Autodesk Inventor part; units mm, degrees
ref_plane "YZ Plane" through (0, 0, 0) normal (1, 0, 0) x (0, 1, 0)
ref_plane "XZ Plane" through (0, 0, 0) normal (0, 1, 0) x (-1, 0, 0)
ref_plane "XY Plane" through (0, 0, 0) normal (0, 0, 1) x (1, 0, 0)
sketch "Esquisse1" plane through (0, 0, 0) normal (0, 0, 1) x (1, 0, 0)
  line L0 (0, 21) -> (40, 21)
  line L1 (40, 21) -> (40, 0)
  line L2 (40, 0) -> (0, 0)
  line L3 (0, 0) -> (0, 21)
  line L4 (-8, 0) -> (48, 0)
  line L5 (0, -4.2) -> (0, 25.2)
  point P0 (0, 0)
  dimension "d0" = 40
  dimension "d1" = 21
extrude "Extrusion1" add sketch "Esquisse1" along normal mid plane 76
sketch "Esquisse2" plane through (0, 0, 38) normal (0, 0, 1) x (1, 0, 0)
  circle A0 centre (10, 10.5) radius 7
  circle A1 centre (30, 10.5) radius 7
  line L0 (40, 21) -> (0, 21)
  line L1 (0, 21) -> (0, 0)
  line L2 (40, 0) -> (40, 21)
  line L3 (0, 0) -> (40, 0)
  dimension "d4" = 14
  dimension "d5" = 14
  dimension "d11" = 10.5
  dimension "d20" = 10.5
  dimension "d21" = 20
extrude "Extrusion2" cut sketch "Esquisse2" against normal through all contours A0 | A1
sketch "Esquisse3" plane through (0, 21, 38) normal (0, 1, 0) x (1, 0, 0)
  line L0 (2, 74) -> (38, 74)
  line L1 (38, 74) -> (38, 2)
  line L2 (38, 2) -> (2, 2)
  line L3 (2, 2) -> (2, 74)
  line L4 (0, 76) -> (40, 76)
  line L5 (40, 0) -> (0, 0)
  line L6 (40, 76) -> (40, 0)
  line L7 (0, 76) -> (0, 0)
  point P0 (0, 38)
  dimension "d14" = 2
  dimension "d15" = 2
  dimension "d16" = 2
  dimension "d17" = 2
extrude "Extrusion3" cut sketch "Esquisse3" against normal blind 14 contours L0 L1 L2 L3
sketch "Esquisse4" plane through (0, 7, 38) normal (0, 1, 0) x (1, 0, 0)
  line L0 (2, 74) -> (19, 74)
  line L1 (19, 74) -> (19, 2)
  line L2 (19, 2) -> (2, 2)
  line L3 (2, 2) -> (2, 74)
  line L4 (20.5, 74) -> (38, 74)
  line L5 (38, 74) -> (38, 2)
  line L6 (38, 2) -> (20.5, 2)
  line L7 (20.5, 2) -> (20.5, 74)
  line L8 (2, 74) -> (38, 74)
  line L9 (2, 2) -> (2, 74)
  line L10 (38, 74) -> (38, 2)
  line L11 (38, 2) -> (2, 2)
  point P0 (0, 38)
  dimension "d22" = 1.5
  dimension "d23" = 17
extrude "Extrusion4" cut sketch "Esquisse4" against normal blind 5 contours L0 L1 L2 L3 | L4 L5 L6 L7
sketch "Esquisse5" plane through (0, 0, 38) normal (0, -1, 0) x (1, 0, 0)
  line L0 (0, 0) -> (40, 0)
  line L1 (0, 0) -> (0, -76)
  line L2 (40, -76) -> (40, 0)
  line L3 (40, -76) -> (0, -76)
  point P0 (0, -38)
  point P1 (10, -10)
  point P2 (10, -38)
  point P3 (30, -38)
  point P4 (30, -66)
  point P5 (30, -10)
  point P6 (10, -66)
  dimension "d26" = 28
  dimension "d27" = 28
  dimension "d28" = 10
  dimension "d29" = 10
  dimension "d30" = 10
  dimension "d31" = 10
  dimension "d32" = 20
  dimension "d33" = 38
  dimension "d41" = 28
  dimension "d42" = 28
  dimension "d43" = 20
hole "Perçage1" at (10, 0, 28) at (10, 0, 0) at (30, 0, 0) at (30, 0, -28) at (10, 0, -28) at (30, 0, 28) direction (0, 1, 0) diameter 2 end through all
equation "\"d5\" = d4"
equation "\"d11\" = d20"
equation "\"d15\" = d14"
equation "\"d16\" = d15"
equation "\"d17\" = d16"
properties part number "support pile"
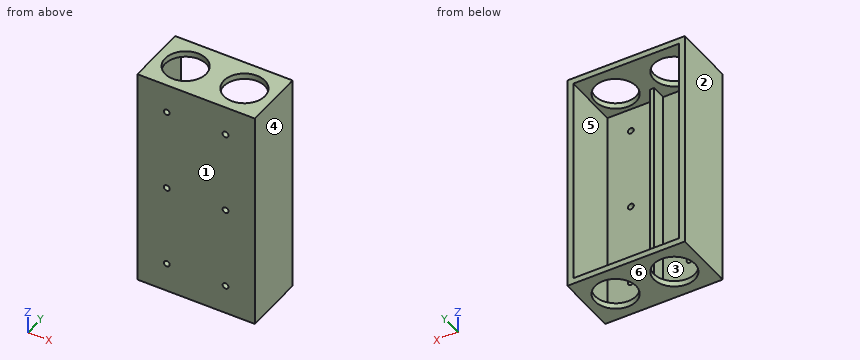
Design review of the part built by this model. Coordinates are the model's own, in mm. Face numbers are marked on the shaded views. A direction names the side the tool comes from. Round coordinates to 2 decimals unless told otherwise and drop trailing zeros. Write each loop counter-clockwise with the first axis right and the second up, starting at its lowest first coordinate (ties: lowest second). Pieces come first, ordered by that corner, then holes.
Item 1: We need section B-B on x = 10. Write out the cut boundary in (y, z).
Item 2: Clearance check with flat-ended pins moving along their axes: pin 1 Ø13.5 at (x, z) = (11, 0) entering from +Y; pin 2 Ø2.5 at (x, z) = (10, 0) entering from -Y; pin 3 Ø19 at (x, z) = (27, 1) entering from +Y. State where each tip first meets the part, or that it passes through.
Item 3: For probe 1 along X at (y, z) = (1.5, -28); probe 2 along X at (y, z) = (5.5, 30.5); probe 3 along Z at (x, y) = (30, 1.25), list the stretches that pass through material, from the lowest coordinate up.
Item 4: We need section A-A on z = 28. Write out the cut boundary in (x, y).
Item 5: We need section D-D on y = 6.25. Write out the cut boundary in (x, z), and give its area (3 significant figures).
Item 6: For the marked faces 5 and 6, list the 3-axis set-ups (+Z, -Z, +X, -X, +Y, -Y) from which the entire face can be reached by the end or side of a thin tool; tool diameter is ignored.
Item 7: We need section C-C on y = 10.5. Write out the cut boundary in (x, z), and give its area (3 significant figures).
Item 8: The part is to be moulded in two halves that separate along X. For the marked faces 1, 2, 3 and 4, say which applies: +X half, -X half, draft (parallel to the pull), parting line (faces both ways), or undercut.
Returned:
1. outline: (0, -38) - (3.5, -38) - (3.5, -36) - (2, -36) - (2, -29) - (0, -29) - close; (0, -27) - (2, -27) - (2, -1) - (0, -1) - close; (0, 1) - (2, 1) - (2, 27) - (0, 27) - close; (0, 29) - (2, 29) - (2, 36) - (3.5, 36) - (3.5, 38) - (0, 38) - close; (17.5, -38) - (21, -38) - (21, -36) - (17.5, -36) - close; (17.5, 36) - (21, 36) - (21, 38) - (17.5, 38) - close
2. pin 1: stops at y = 2
2. pin 2: stops at y = 0
2. pin 3: stops at y = 7
3. probe 1: x = 0 to 9, 11 to 29, 31 to 40
3. probe 2: x = 0 to 2, 19 to 20.5, 38 to 40
3. probe 3: z = -38 to -29, -27 to -1, 1 to 27, 29 to 38
4. outline: (0, 0) - (9, 0) - (9, 2) - (2, 2) - (2, 21) - (0, 21) - close; (11, 0) - (29, 0) - (29, 2) - (20.5, 2) - (20.5, 7) - (19, 7) - (19, 2) - (11, 2) - close; (31, 0) - (40, 0) - (40, 21) - (38, 21) - (38, 2) - (31, 2) - close
5. outline: (0, -38) - (4.44, -38) - (4.44, -36) - (2, -36) - (2, 36) - (4.44, 36) - (4.44, 38) - (0, 38) - close; (15.56, -38) - (24.44, -38) - (24.44, -36) - (20.5, -36) - (20.5, 36) - (24.44, 36) - (24.44, 38) - (15.56, 38) - (15.56, 36) - (19, 36) - (19, -36) - (15.56, -36) - close; (35.56, -38) - (40, -38) - (40, 38) - (35.56, 38) - (35.56, 36) - (38, 36) - (38, -36) - (35.56, -36) - close
5. area: 467 mm2
6. face 5: +Y
6. face 6: -Z, +X, -X, +Y, -Y
7. outline: (0, -38) - (3, -38) - (3, -36) - (2, -36) - (2, 36) - (3, 36) - (3, 38) - (0, 38) - close; (17, -38) - (23, -38) - (23, -36) - (17, -36) - close; (17, 36) - (23, 36) - (23, 38) - (17, 38) - close; (37, -38) - (40, -38) - (40, 38) - (37, 38) - (37, 36) - (38, 36) - (38, -36) - (37, -36) - close
7. area: 336 mm2
8. face 1: draft
8. face 2: -X half
8. face 3: undercut
8. face 4: +X half
